```python
from build123d import *

# Parameters (mm, degrees)
SKETCH020_W                   = 95
SKETCH020_H                   = 82
PAD005_DEPTH                  = 3
SKETCH021_W                   = 11
SKETCH021_H                   = 3
SKETCH021_W_2                 = 16
SKETCH021_W_3                 = 3
SKETCH021_H_2                 = 14.5
SKETCH021_H_3                 = 11
POCKET015_DEPTH               = 254.062745
SKETCH021_MIRRORED019_2_W     = 11
SKETCH021_MIRRORED019_2_H     = 3
SKETCH021_MIRRORED019_2_W_2   = 16
SKETCH021_MIRRORED019_2_W_3   = 3
SKETCH021_MIRRORED019_2_H_2   = 14.5
SKETCH021_MIRRORED019_2_H_3   = 11
POCKET015_MIRRORED019_2_DEPTH = 254.062745
SKETCH022_W                   = 4
SKETCH022_H                   = 2.5
POCKET016_DEPTH               = 254.062745
POCKET017_DEPTH               = 3.001
SKETCH022_MIRRORED026_2_W     = 4
SKETCH022_MIRRORED026_2_H     = 2.5
POCKET016_MIRRORED026_2_DEPTH = 254.062745


with BuildPart() as part:
    # Sketch020 → Pad005 (new body)
    with BuildSketch(Plane.YZ):
        Rectangle(SKETCH020_W, SKETCH020_H)
    extrude(amount=PAD005_DEPTH)

    # Sketch021 → Pocket015 (cut, through all)
    with BuildSketch(Plane.YZ):
        with Locations((0, 39.5)):
            Rectangle(SKETCH021_W, SKETCH021_H)
        with Locations((-33.5, 39.5)):
            Rectangle(SKETCH021_W_2, SKETCH021_H)
        with Locations((33.5, 39.5)):
            Rectangle(SKETCH021_W_2, SKETCH021_H)
        with Locations((-46, 30.75)):
            Rectangle(SKETCH021_W_3, SKETCH021_H_2)
        with Locations((-46, 0)):
            Rectangle(SKETCH021_W_3, SKETCH021_H_3)
    pocket015 = extrude(amount=POCKET015_DEPTH, mode=Mode.SUBTRACT)

    # Sketch021 Mirrored019 2 → Pocket015 Mirrored019 2 (cut, through all)
    with BuildSketch(Plane(origin=(0, 0, 0), x_dir=(0, 1, 0), z_dir=(-1, 0, 0))):
        with Locations((0, 39.5)):
            Rectangle(SKETCH021_MIRRORED019_2_W, SKETCH021_MIRRORED019_2_H)
        with Locations((-33.5, 39.5)):
            Rectangle(SKETCH021_MIRRORED019_2_W_2, SKETCH021_MIRRORED019_2_H)
        with Locations((33.5, 39.5)):
            Rectangle(SKETCH021_MIRRORED019_2_W_2, SKETCH021_MIRRORED019_2_H)
        with Locations((-46, 30.75)):
            Rectangle(SKETCH021_MIRRORED019_2_W_3, SKETCH021_MIRRORED019_2_H_2)
        with Locations((-46, 0)):
            Rectangle(SKETCH021_MIRRORED019_2_W_3, SKETCH021_MIRRORED019_2_H_3)
    pocket015_mirrored019_2 = extrude(amount=-POCKET015_MIRRORED019_2_DEPTH, mode=Mode.SUBTRACT)

    # Mirrored028: Pocket015, Pocket015 Mirrored019 2 across Sketch021 V_Axis
    add(pocket015.mirror(Plane(origin=(0, 0, 0), x_dir=(1, 0, 0), z_dir=(0, 1, 0))), mode=Mode.SUBTRACT)
    add(pocket015_mirrored019_2.mirror(Plane(origin=(0, 0, 0), x_dir=(1, 0, 0), z_dir=(0, 1, 0))), mode=Mode.SUBTRACT)

    # Sketch022 → Pocket016 (cut, through all)
    with BuildSketch(Plane.YZ):
        Polygon((-32.25, 41), (-32.25, 32), (-31, 32), (-31, 30), (-32.25, 30), (-32.25, 27), (-34.75, 27), (-34.75, 30), (-36, 30), (-36, 32), (-34.75, 32), (-34.75, 41), align=None)
        with Locations((-45.5, 14.5)):
            Rectangle(SKETCH022_W, SKETCH022_H)
    pocket016 = extrude(amount=POCKET016_DEPTH, mode=Mode.SUBTRACT)

    # Sketch023 → Pocket017 (cut, through all)
    with BuildSketch(Plane.YZ):
        with BuildLine():
            Line((-20.5, 5), (24.5, 5))
            ThreePointArc((24.5, 5), (26.62132, 5.87868), (27.5, 8))
            Line((27.5, 8), (27.5, 32))
            ThreePointArc((27.5, 32), (26.62132, 34.12132), (24.5, 35))
            Line((24.5, 35), (-20.5, 35))
            ThreePointArc((-20.5, 35), (-22.62132, 34.12132), (-23.5, 32))
            Line((-23.5, 32), (-23.5, 8))
            ThreePointArc((-23.5, 8), (-22.62132, 5.87868), (-20.5, 5))
        make_face()
        with BuildLine():
            ThreePointArc((-13, 0), (-27.5, -14.5), (-13, -29))
            Line((-13, -29), (13, -29))
            ThreePointArc((13, -29), (27.5, -14.5), (13, 0))
            Line((-13, 0), (13, 0))
        make_face()
    extrude(amount=POCKET017_DEPTH, mode=Mode.SUBTRACT)

    # Sketch022 Mirrored026 2 → Pocket016 Mirrored026 2 (cut, through all)
    with BuildSketch(Plane(origin=(0, 0, 0), x_dir=(0, -1, 0), z_dir=(-1, 0, 0))):
        Polygon((-32.25, 41), (-32.25, 32), (-31, 32), (-31, 30), (-32.25, 30), (-32.25, 27), (-34.75, 27), (-34.75, 30), (-36, 30), (-36, 32), (-34.75, 32), (-34.75, 41), align=None)
        with Locations((-45.5, 14.5)):
            Rectangle(SKETCH022_MIRRORED026_2_W, SKETCH022_MIRRORED026_2_H)
    pocket016_mirrored026_2 = extrude(amount=-POCKET016_MIRRORED026_2_DEPTH, mode=Mode.SUBTRACT)

    # Mirrored027: Pocket016, Pocket016 Mirrored026 2 across Sketch022 H_Axis
    add(pocket016.mirror(Plane.XY), mode=Mode.SUBTRACT)
    add(pocket016_mirrored026_2.mirror(Plane.XY), mode=Mode.SUBTRACT)


with BuildPart() as part_1:
    # Body005 placement: moved
    add(part.part.moved(Location((57, 0, 0))))


solid = part_1.part
```
The listing builds one solid part. Answer for the finished solid, in the listing's coordinates (mm). A direction names the side the tool comes from. Coordinates: 2 decimals unless noted, no trailing zeros. Write each loop counter-clockwise with the first axis right and the second up, starting at its lowest first coordinate (ties: lowest second). Pieces come first, ordered by that corner, then holes. Notation, with made-up numbers: (2.5, 25) -> (34.5, 25) arc R21 cw to (34.5, 52) -> close; hole circle Ø2 at (15, 48). An arc over 180 degrees is marked (long way). Write each question's results on one line, items separated by ' | '. Start each with the question number.
1) A tool of negligible diameter and unlimited length cuts with its end or side. For faces 1 (the flat face through (58, -32.25, -29)), 2 (the cylindrical face through (58.479, 27.496, -14.819)), 3 (the flat face through (58, -44.5, 31)), 4 (the flat face through (58, 32.25, 29)), from which of +Z, -Z, +X, -X, +Y, -Y can it reach the whole face along a straight path? Write none if from no direction.
2) For a pull along Y with two mould halves and no side action, classify faces 5 (the flat face through (58, -46, 13.25)), 6 (the flat face through (58, -47.5, 39)), 7 (the flat face through (58, 36, 31)) as +Y half, -Y half, draft (parallel to the pull), parting line (faces both ways), or undercut.
3) A cutting plane is placed at C-C (y = -8.5). Determine the outline of the cut face in (x, z), then the cut area to 3 significant figures.
4) Straight lines are drawn through the part: probe 1 along Z at (x, y) = (59.6, -7.5); probe 2 along Z at (x, y) = (58.7, -3.5); probe 3 along Y at (x, z) = (57.1, 37.5). For each, find the intervals that lie inside material, in ascending order.
5) Flat-ended cylindrical pins translate along their axes: pin 1 Ø1.5 at (x, y) = (58.5, -3) entering from -Z; pin 2 Ø1 at (x, z) = (58.5, 31) entering from -Y; pin 3 Ø1 at (x, z) = (58, 31) entering from +Y. Find the tip coordinate at first contact, or state that the pin passes through.
6) A cutting plane is placed at D-D (x = 57.45). Count the separate pieces of the cut face and the enclosed holes in it, then the cut area to 3 significant figures.
7) A cutting plane is placed at A-A (y = 1). Determine the outline of the cut face in (x, z).
8) A cutting plane is placed at B-B (z = -14.5). Determine the outline of the cut face in (x, y), then the cut area to 3 significant figures.
Values follow:
1) face 1: -Z, +X, -X | face 2: +X, -X | face 3: +X, -X, -Y | face 4: +Z, +X, -X
2) face 5: draft | face 6: -Y half | face 7: undercut
3) outline: (57, -41) -> (60, -41) -> (60, -29) -> (57, -29) -> close; (57, 0) -> (60, 0) -> (60, 5) -> (57, 5) -> close; (57, 35) -> (60, 35) -> (60, 41) -> (57, 41) -> close | area: 69.0 mm²
4) probe 1: -41 to -29, 0 to 5, 35 to 41 | probe 2: -38 to -29, 0 to 5, 35 to 38 | probe 3: -44.5 to -34.75, -32.25 to 32.25, 34.75 to 44.5
5) pin 1: z = -38 | pin 2: y = -44.5 | pin 3: y = 44.5
6) separate pieces: 1 | enclosed holes: 2 | area: 4,190 mm²
7) outline: (57, -38) -> (60, -38) -> (60, -29) -> (57, -29) -> close; (57, 0) -> (60, 0) -> (60, 5) -> (57, 5) -> close; (57, 35) -> (60, 35) -> (60, 38) -> (57, 38) -> close
8) outline: (57, -43.5) -> (60, -43.5) -> (60, -27.5) -> (57, -27.5) -> close; (57, 27.5) -> (60, 27.5) -> (60, 43.5) -> (57, 43.5) -> close | area: 96.0 mm²
